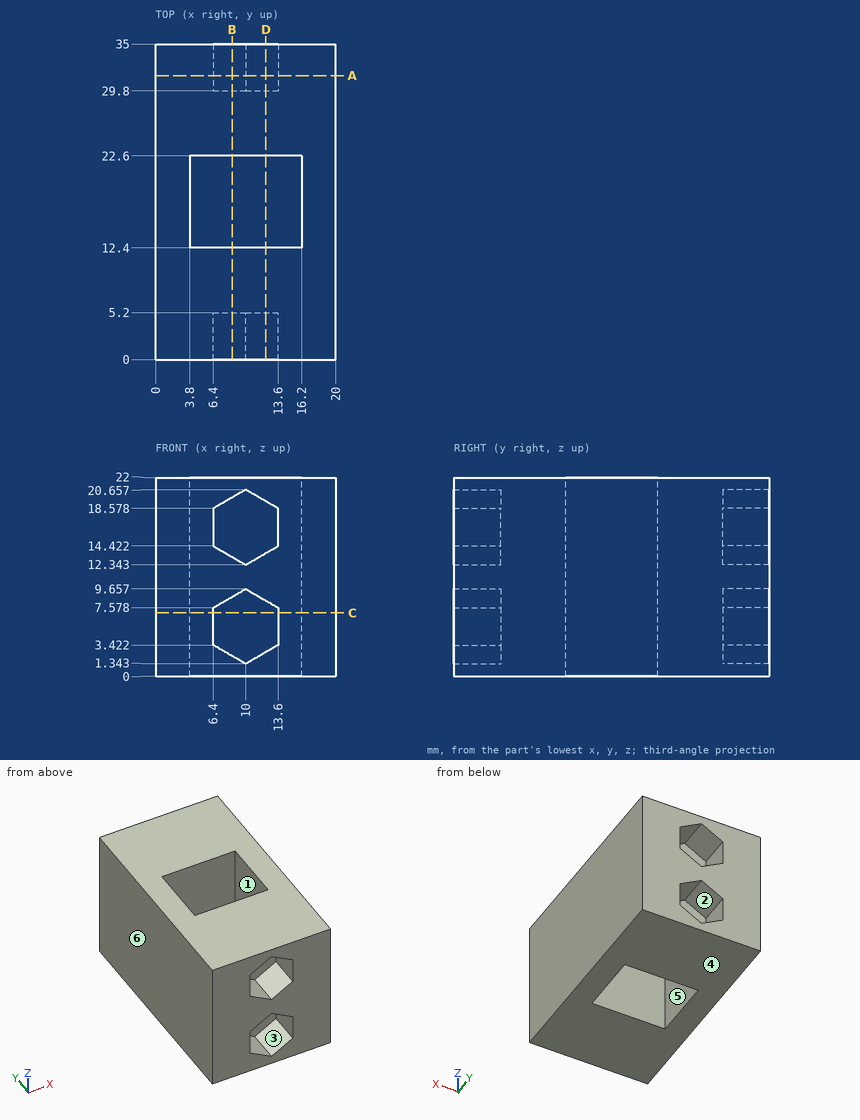
Source: three-view drawing plus pictorial views. Frame: mm from the lowest corner of the part. A direction names the side the tool comes from. Round coordinates to 2 decimals unless told otherwise and drop trailing zeros. Loops run counter-clockwise (first coordinate to the right, second up) from the corner with the lowest first, then second, coordinate; pieces in that order, holes last. Notation, with made-up numbers: M 71.5,25 L 106.5,25 A26 cw 106.5,41 Z; hole C 52,79 d7. An arc over 180 degrees is marked long. Answer as CSV lines item,"result". Start each with the question number.
(1) First-contact query: pin 1 (3.5 mm diameter, centred on x = 9.5, z = 16.5, fed in from -Y); pin 2 (2 mm diameter, centred on x = 10, z = 4.5, fed in from +Y). Flat tips, straight axial feed; report the tip coordinate or a pass-through.
(2) Section C-C, the plane z = 7. Output: boundary loops of the cut face in (x, y).
(3) Section A-A, the plane y = 31.5. Output: boundary loops of the cut face in (x, z).
(4) Section B-B, the plane x = 8.5. Output: boundary loops of the cut face in (y, z).
(5) Line query: line 1 (Y direction, x = 10.75, z = 19.75); line 2 (X direction, y = 14.5, z = 7.25); line 3 (Y direction, x = 13.25, z = 13). Output: solid intervals per line, ascending. Write a range as [from, to].
(6) Draft query along X for the marked faces 4, 5 and 6. Return one class per face: released by +X, released by -X, zero draft, split by the parting line, or undercut.
(7) Reachability of the marked faces 1, 2 and 3 from +Z, -Z, +X, -X, +Y, -Y: full face, straight path, thin tool, end or side. Return the list, or none.
(8) Section D-D, the plane x = 12.25. Output: boundary loops of the cut face in (y, z).
Values found:
1,pin 1,"stops at y = 5.2"
1,pin 2,"stops at y = 29.8"
2,outline,"M 0,0 L 6.4,0 L 6.4,5.2 L 13.6,5.2 L 13.6,0 L 20,0 L 20,35 L 13.6,35 L 13.6,29.8 L 6.4,29.8 L 6.4,35 L 0,35 Z; hole M 3.8,12.4 L 16.2,12.4 L 16.2,22.6 L 3.8,22.6 Z"
3,outline,"M 0,0 L 20,0 L 20,22 L 0,22 Z; hole M 6.4,3.42 L 10,1.34 L 13.6,3.42 L 13.6,7.58 L 10,9.66 L 6.4,7.58 Z; hole M 6.4,14.42 L 10,12.34 L 13.6,14.42 L 13.6,18.58 L 10,20.66 L 6.4,18.58 Z"
4,outline,"M 0,0 L 12.4,0 L 12.4,22 L 0,22 L 0,19.79 L 5.2,19.79 L 5.2,13.21 L 0,13.21 L 0,8.79 L 5.2,8.79 L 5.2,2.21 L 0,2.21 Z; M 22.6,0 L 35,0 L 35,2.21 L 29.8,2.21 L 29.8,8.79 L 35,8.79 L 35,13.21 L 29.8,13.21 L 29.8,19.79 L 35,19.79 L 35,22 L 22.6,22 Z"
5,line 1,"y = [5.2, 12.4], [22.6, 29.8]"
5,line 2,"x = [0, 3.8], [16.2, 20]"
5,line 3,"y = [0, 12.4], [22.6, 35]"
6,face 4,"zero draft"
6,face 5,"undercut"
6,face 6,"released by -X"
7,face 1,"+Z, -Z"
7,face 2,"+Y"
7,face 3,"-Y"
8,outline,"M 0,0 L 12.4,0 L 12.4,22 L 0,22 L 0,19.36 L 5.2,19.36 L 5.2,13.64 L 0,13.64 L 0,8.36 L 5.2,8.36 L 5.2,2.64 L 0,2.64 Z; M 22.6,0 L 35,0 L 35,2.64 L 29.8,2.64 L 29.8,8.36 L 35,8.36 L 35,13.64 L 29.8,13.64 L 29.8,19.36 L 35,19.36 L 35,22 L 22.6,22 Z"
